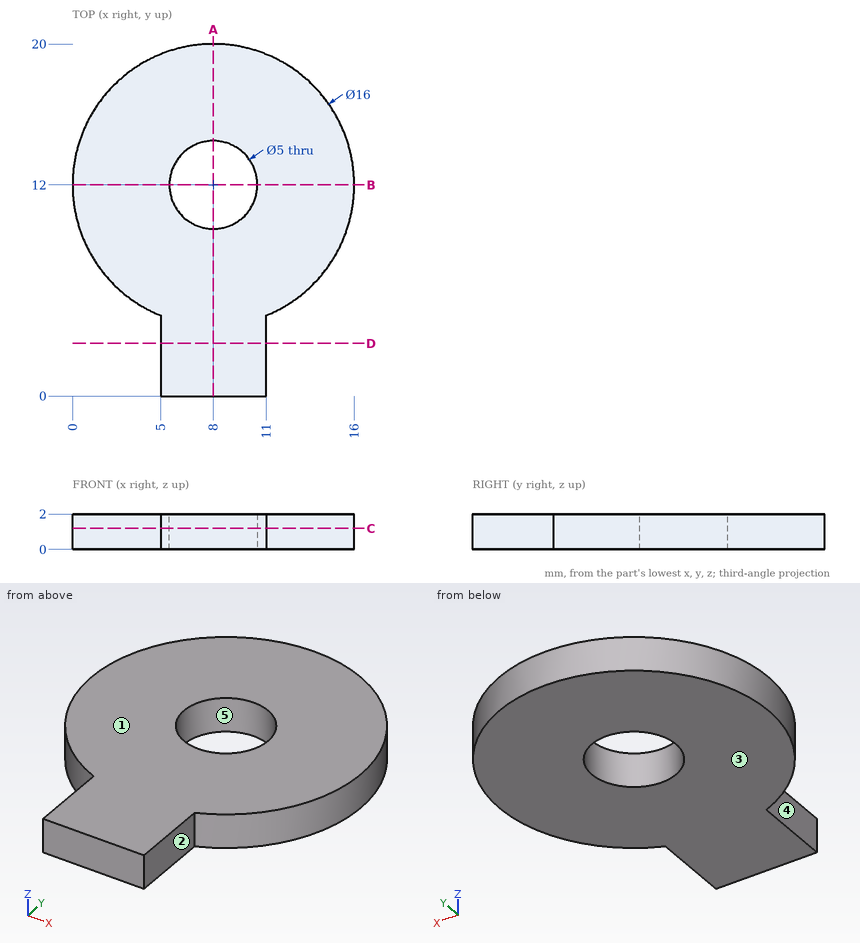
Part print with two shaded views. Sizes in mm from the minimum x, y, z corner. A direction names the side the tool comes from. Round coordinates to 2 decimals unless told otherwise and drop trailing zeros. Loops run counter-clockwise (first coordinate to the right, second up) from the corner with the lowest first, then second, coordinate; pieces in that order, holes last. Notation, with made-up numbers: M -27.5,18 L 29.5,18 A15 cw 29.5,31 Z; hole C -39,54.25 d11. An arc over 180 degrees is marked long. Put each result on its own line as item: value. Start each with the question number.
Item 1: Cut at B-B (y = 12). List the corners of the cut face in (x, z).
Item 2: Cut at D-D (y = 3). List the corners of the cut face in (x, z), then the cut area to 3 significant figures.
Item 3: Cut at C-C (z = 1.2). List the corners of the cut face in (x, y), then the cut area to 3 significant figures.
Item 4: 3-axis set-ups, long thin cutter, end or side, ignore diameter. For the marked faces 1 and 2: which of +Z, -Z, +X, -X, +Y, -Y reach the whole face in a straight line?
Item 5: Cut at A-A (x = 8). List the corners of the cut face in (y, z).
Item 6: Drill centre lines: line 1 along Y through (x, z) = (8, 0.5); line 2 along Y through (x, z) = (5.75, 1.65); line 3 along X through (y, z) = (13.5, 0.55). Where is each one in solid material? Low to high.
Item 7: Drop a flat-ended pin along its axis: P1, Ø4.5, axis at x = 8, y = 12, coming from the +Z side. Give the stop position or say it passes through.
Item 8: Mould opens along X. For the marked faces 3, 4 and 5 say: released by +X, released by -X, zero draft, split by the parting line, or undercut.
Answer block:
1. outline: M 0,0 L 5.5,0 L 5.5,2 L 0,2 Z; M 10.5,0 L 16,0 L 16,2 L 10.5,2 Z
2. outline: M 5,0 L 11,0 L 11,2 L 5,2 Z
2. area: 12.0 mm2
3. outline: M 5,0 L 11,0 L 11,4.58 A8 ccw long 5,4.58 Z; hole C 8,12 d5
3. area: 207 mm2
4. face 1: +Z, +X, -X, +Y, -Y
4. face 2: +Z, -Z, +X, -Y
5. outline: M 0,0 L 9.5,0 L 9.5,2 L 0,2 Z; M 14.5,0 L 20,0 L 20,2 L 14.5,2 Z
6. line 1: 0 to 9.5, 14.5 to 20
6. line 2: 0 to 10.91, 13.09 to 19.68
6. line 3: 0.14 to 6, 10 to 15.86
7. P1: through
8. face 3: zero draft
8. face 4: released by -X
8. face 5: undercut
